```python
from build123d import *

# Parameters (mm, degrees)
BOSS_EXTRUDE1_DEPTH     = 4.064
SKETCH14_W              = 9.017
SKETCH14_H              = 2.54
BOSS_EXTRUDE5_DEPTH     = 1.27
SKETCH15_W              = 1.905
SKETCH15_H              = 2.54
BOSS_EXTRUDE6_DEPTH     = 0.508
SKETCH16_W              = 1.016
SKETCH16_H              = 2.54
BOSS_EXTRUDE7_DEPTH     = 3.175
SKETCH17_R              = 0.75565
CUT_EXTRUDE6_DEPTH      = 3.175
SKETCH18_R              = 0.381
CUT_EXTRUDE7_DEPTH      = 3.175
CUT_EXTRUDE9_DEPTH      = 11.204992749
CUT_EXTRUDE9_DEPTH_BACK = 2.54
SKETCH19_R              = 0.5969
SKETCH20_R              = 0.75565
CUT_EXTRUDE10_DEPTH     = 10


with BuildPart() as part:
    # Sketch1 → Boss-Extrude1 (new body)
    with BuildSketch(Plane.XY):
        Polygon((0, 0), (-2.45, 0), (-2.45, 1.778), (0, 1.778), (0, 4.826), (-2.45, 4.826), (-2.45, 6.604), (0, 6.604), (1.27, 6.604), (2.54, 5.334), (2.54, 1.27), (1.27, 0), align=None)
    extrude(amount=BOSS_EXTRUDE1_DEPTH)

    # Sketch14 → Boss-Extrude5 (add)
    with BuildSketch(Plane(origin=(2.54, 0, 0), x_dir=(0, 0, -1), z_dir=(1, 0, 0))):
        with Locations((-1.4605, 3.302)):
            Rectangle(SKETCH14_W, SKETCH14_H)
    extrude(amount=BOSS_EXTRUDE5_DEPTH)

    # Sketch15 → Boss-Extrude6 (add)
    with BuildSketch(Plane.ZY.offset(-2.54)):
        with Locations((5.0165, 3.302)):
            Rectangle(SKETCH15_W, SKETCH15_H)
    extrude(amount=BOSS_EXTRUDE6_DEPTH)

    # Sketch16 → Boss-Extrude7 (add)
    with BuildSketch(Plane(origin=(3.81, 0, 0), x_dir=(0, 0, -1), z_dir=(1, 0, 0))):
        with Locations((2.54, 3.302)):
            Rectangle(SKETCH16_W, SKETCH16_H)
    extrude(amount=BOSS_EXTRUDE7_DEPTH)

    # Sketch17 → Cut-Extrude6 (cut)
    with BuildSketch(Plane(origin=(0, 0, -3.048), x_dir=(-1, 0, 0), z_dir=(0, 0, -1))):
        with Locations((-5.3975, 3.302)):
            Circle(SKETCH17_R)
    extrude(amount=-CUT_EXTRUDE6_DEPTH, mode=Mode.SUBTRACT)

    # Sketch18 → Cut-Extrude7 (cut)
    with BuildSketch(Plane.XZ.offset(-2.032)):
        with Locations((2.921, 4.953)):
            Circle(SKETCH18_R)
    extrude(amount=-CUT_EXTRUDE7_DEPTH, mode=Mode.SUBTRACT)

    # Sketch19 → Cut-Extrude9 (cut, two sides: drawn at the far end of the back side and taken through both)
    with BuildSketch(Plane(origin=(2.54, 0, 0), x_dir=(0, 0, -1), z_dir=(1, 0, 0)).offset(-CUT_EXTRUDE9_DEPTH_BACK)):
        with Locations((-2.032, 4.572)):
            Circle(SKETCH19_R)
        with Locations(Location((-2.032, 2.032, 0), (0, 0, 334.815663466))):
            Circle(SKETCH19_R)
    extrude(amount=CUT_EXTRUDE9_DEPTH + CUT_EXTRUDE9_DEPTH_BACK, mode=Mode.SUBTRACT)

    # Sketch20 → Cut-Extrude10 (cut)
    with BuildSketch(Plane(origin=(0, 6.604, 0), x_dir=(1, 0, 0), z_dir=(0, 1, 0))):
        with Locations(Location((-1.18, -2.032, 0), (0, 0, 180))):
            Circle(SKETCH20_R)
    extrude(amount=-CUT_EXTRUDE10_DEPTH, mode=Mode.SUBTRACT)


solid = part.part
```
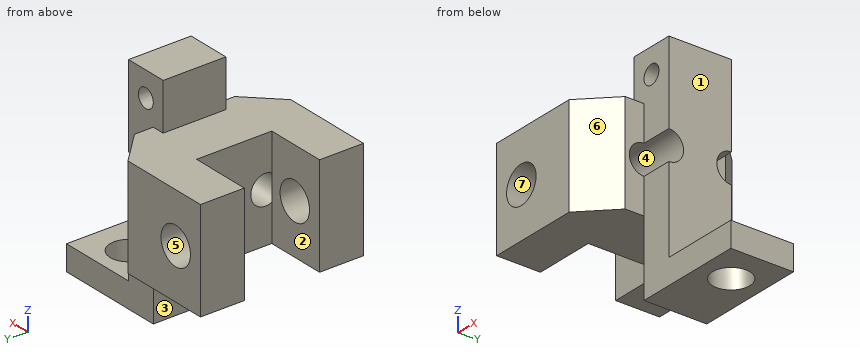
Input: part model. Units: mm. Frame: model coordinates. Face numbers are marked on the shaded views. A direction names the side the tool comes from. Round coordinates to 2 decimals unless told otherwise and drop trailing zeros. Loops run counter-clockwise (first coordinate to the right, second up) from the corner with the lowest first, then second, coordinate; pieces in that order, holes last.
1) Section query C-C on x = 5.5. Return the cut outline in (y, z).
Ans:
outline: (2.03, -3.05) - (2.55, -3.05) - (2.55, -2.03) - (2.03, -2.03) - close; (4.05, -3.05) - (4.57, -3.05) - (4.57, -2.03) - (4.05, -2.03) - close
2) Section query A-A on x = -1.18. Return the cut outline in (y, z).
Ans:
outline: (0, 0) - (1.78, 0) - (1.78, 1.28) - (0, 1.28) - close; (0, 2.79) - (1.78, 2.79) - (1.78, 4.06) - (0, 4.06) - close; (4.83, 0) - (6.6, 0) - (6.6, 1.28) - (4.83, 1.28) - close; (4.83, 2.79) - (6.6, 2.79) - (6.6, 4.06) - (4.83, 4.06) - close
3) Section query D-D on z = 0.75. Return the cut outline in (x, y), plus the area to 3 significant figures.
Ans:
outline: (-2.45, 0) - (1.27, 0) - (2.54, 1.27) - (2.54, 2.03) - (3.81, 2.03) - (3.81, 4.57) - (2.54, 4.57) - (2.54, 5.33) - (1.27, 6.6) - (-2.45, 6.6) - (-2.45, 4.83) - (0, 4.83) - (0, 1.78) - (-2.45, 1.78) - close
area: 27.1 mm2
4) Set-up query: the marked faces 1, 2 and 3. Return all of +Z, -Z, +X, -X, +Y, -Y with unobstructed straight access to the full face (end or side cutting, diameter ignored); none if empty.
Ans:
face 1: +Z, +X, +Y, -Y
face 2: +Z, -Z, -X
face 3: -Z, -X, +Y, -Y
5) Pin query (flat end, axial travel): pin 1 (0.6 mm diameter, centred on y = 3, z = 5, fed in from -X); pin 2 (2 mm diameter, centred on x = 4, z = 0, fed in from +Y); pin 3 (1.4 mm diameter, centred on x = 3, z = 4.5, fed in from -Y). Return the tip coordinate at first contact, or that it passes through.
Ans:
pin 1: stops at x = 2.03
pin 2: stops at y = 4.57
pin 3: stops at y = 1.18
6) Material intervals for line 1 (Z direction, x = -1.18, y = 6.15); line 2 (X direction, y = 4, z = 5); line 3 (Z direction, x = 6.75, y = 3.5), sorted ascending.
Ans:
line 1: z = 0 to 1.28, 2.79 to 4.06
line 2: x = 2.03 to 2.54, 3.3 to 3.81
line 3: z = -3.05 to -2.03
7) Pull-direction query (X, two-part tool) for the marked faces 4, 5, 6 and 7; classes: released by +X, released by -X, zero draft, split by the parting line, or undercut.
Ans:
face 4: zero draft
face 5: undercut
face 6: released by +X
face 7: undercut
8) Section query B-B on z = 4.75. Return the cut outline in (x, y), plus the area to 3 significant figures.
Ans:
outline: (2.03, 2.03) - (2.6, 2.03) - (2.6, 4.57) - (2.03, 4.57) - close; (3.24, 2.03) - (3.81, 2.03) - (3.81, 4.57) - (3.24, 4.57) - close
area: 2.88 mm2
